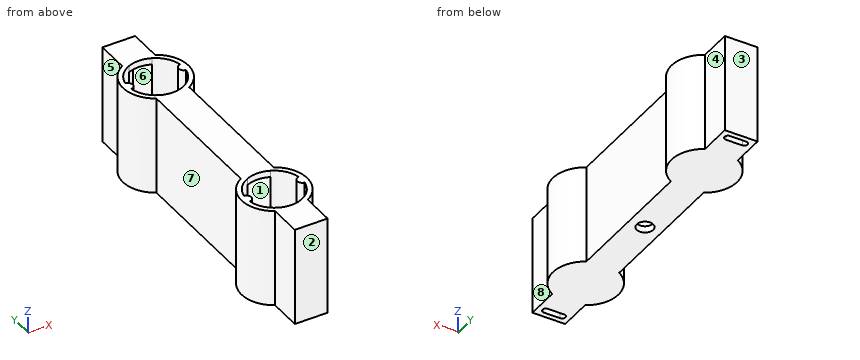
from build123d import *
from build123d.topology import SkipClean

# Parameters (mm, degrees)
BOSS_EXTRU_1_DEPTH      = 30
ENL_V_MAT_EXTRU_1_DEPTH = 28
BOSS_EXTRU_2_DEPTH      = 2
ESQUISSE5_R             = 2.5
ENL_V_MAT_EXTRU_2_DEPTH = 2
BOSS_EXTRU_3_DEPTH      = 29
ENL_V_MAT_EXTRU_4_DEPTH = 29
BOSS_EXTRU_4_DEPTH      = 28


with BuildPart() as part:
    # Esquisse1 → Boss.-Extru.1 (new body)
    with BuildSketch(Plane.XY):
        with BuildLine():
            Line((-5, -21.339745962), (-5, 21.339745962))
            ThreePointArc((-5, 21.339745962), (-10, 30), (-5, 38.660254038))
            Line((-5, 38.660254038), (-5, 48.660254038))
            Line((-5, 48.660254038), (5, 48.660254038))
            Line((5, 48.660254038), (5, 38.660254038))
            ThreePointArc((5, 38.660254038), (10, 30), (5, 21.339745962))
            Line((5, 21.339745962), (5, -21.339745962))
            ThreePointArc((5, -21.339745962), (10, -30), (5, -38.660254038))
            Line((5, -38.660254038), (5, -48.660254038))
            Line((5, -48.660254038), (-5, -48.660254038))
            Line((-5, -48.660254038), (-5, -38.660254038))
            ThreePointArc((-5, -38.660254038), (-10, -30), (-5, -21.339745962))
        make_face()
    extrude(amount=BOSS_EXTRU_1_DEPTH)

    # Esquisse2 → Enl_v. mat.-Extru.1 (cut)
    with BuildSketch(Plane.XY.offset(30)):
        with BuildLine():
            Line((-3.5, 22.254033308), (-3.5, -22.254033308))
            ThreePointArc((-3.5, -22.254033308), (-8.5, -30), (-3.5, -37.745966692))
            Line((-3.5, -37.745966692), (-3.5, -47.160254038))
            Line((-3.5, -47.160254038), (3.5, -47.160254038))
            Line((3.5, -47.160254038), (3.5, -37.745966692))
            ThreePointArc((3.5, -37.745966692), (8.5, -30), (3.5, -22.254033308))
            Line((3.5, -22.254033308), (3.5, 22.254033308))
            ThreePointArc((3.5, 22.254033308), (8.5, 30), (3.5, 37.745966692))
            Line((3.5, 37.745966692), (3.5, 47.160254038))
            Line((3.5, 47.160254038), (-3.5, 47.160254038))
            Line((-3.5, 47.160254038), (-3.5, 37.745966692))
            ThreePointArc((-3.5, 37.745966692), (-8.5, 30), (-3.5, 22.254033308))
        make_face()
    extrude(amount=-ENL_V_MAT_EXTRU_1_DEPTH, mode=Mode.SUBTRACT)

    # Esquisse3 → Boss.-Extru.2 (add)
    with SkipClean():  # keep this step's faces unmerged: merging them makes the solid invalid here
        with BuildSketch(Plane.XY.offset(30)):
            with BuildLine():
                Line((-3.5, 37.745966692), (-3.5, 47.160254038))
                Line((-3.5, 47.160254038), (3.5, 47.160254038))
                Line((3.5, 47.160254038), (3.5, 37.745966692))
                ThreePointArc((3.5, 37.745966692), (0, 38.5), (-3.5, 37.745966692))
            make_face()
            with BuildLine():
                Line((-3.5, -37.745966692), (-3.5, -47.160254038))
                Line((-3.5, -47.160254038), (3.5, -47.160254038))
                Line((3.5, -47.160254038), (3.5, -37.745966692))
                ThreePointArc((3.5, -37.745966692), (0, -38.5), (-3.5, -37.745966692))
            make_face()
            with BuildLine():
                Line((3.5, -22.254033308), (3.5, 22.254033308))
                ThreePointArc((3.5, 22.254033308), (0, 21.5), (-3.5, 22.254033308))
                Line((-3.5, 22.254033308), (-3.5, -22.254033308))
                ThreePointArc((-3.5, -22.254033308), (0, -21.5), (3.5, -22.254033308))
            make_face()
        extrude(amount=-BOSS_EXTRU_2_DEPTH)

    # Esquisse5 → Enl_v. mat.-Extru.2 (cut)
    with SkipClean():  # keep this step's faces unmerged: merging them makes the solid invalid here
        with BuildSketch(Plane(origin=(0, 0, 0), x_dir=(-1, 0, 0), z_dir=(0, 0, -1))):
            Circle(ESQUISSE5_R)
            with BuildLine():
                Line((2.5, 45.074057395), (-2.5, 45.074057395))
                ThreePointArc((-2.5, 45.074057395), (-3.5, 46.074057395), (-2.5, 47.074057395))
                Line((-2.5, 47.074057395), (2.5, 47.074057395))
                ThreePointArc((2.5, 47.074057395), (3.5, 46.074057395), (2.5, 45.074057395))
            make_face()
            with BuildLine():
                Line((2.5, -45.074057395), (-2.5, -45.074057395))
                ThreePointArc((-2.5, -45.074057395), (-3.5, -46.074057395), (-2.5, -47.074057395))
                Line((-2.5, -47.074057395), (2.5, -47.074057395))
                ThreePointArc((2.5, -47.074057395), (3.5, -46.074057395), (2.5, -45.074057395))
            make_face()
        extrude(amount=-ENL_V_MAT_EXTRU_2_DEPTH, mode=Mode.SUBTRACT)

    # Esquisse8 → Boss.-Extru.3 (add)
    with SkipClean():  # keep this step's faces unmerged: merging them makes the solid invalid here
        with BuildSketch(Plane.XY.offset(30)):
            with BuildLine():
                ThreePointArc((8.367647059, -28.50585051), (7, -30), (8.367647059, -31.49414949))
                ThreePointArc((8.367647059, -31.49414949), (0, -38.5), (-8.367647059, -31.49414949))
                ThreePointArc((-8.367647059, -31.49414949), (-7, -30), (-8.367647059, -28.50585051))
                ThreePointArc((-8.367647059, -28.50585051), (0, -21.5), (8.367647059, -28.50585051))
            make_face()
        extrude(amount=-BOSS_EXTRU_3_DEPTH)

    # Esquisse8_15 → Enl_v. mat.-Extru.4 (cut)
    with SkipClean():  # keep this step's faces unmerged: merging them makes the solid invalid here
        with BuildSketch(Plane.XY.offset(30)):
            with BuildLine():
                ThreePointArc((-3.5, -37.745966692), (0, -38.5), (3.5, -37.745966692))
                ThreePointArc((3.5, -37.745966692), (6.706829822, -35.221918588), (8.367647059, -31.49414949))
                ThreePointArc((8.367647059, -31.49414949), (7, -30), (8.367647059, -28.50585051))
                ThreePointArc((8.367647059, -28.50585051), (6.706829822, -24.778081412), (3.5, -22.254033308))
                ThreePointArc((3.5, -22.254033308), (0, -21.5), (-3.5, -22.254033308))
                ThreePointArc((-3.5, -22.254033308), (-6.706829822, -24.778081412), (-8.367647059, -28.50585051))
                ThreePointArc((-8.367647059, -28.50585051), (-7, -30), (-8.367647059, -31.49414949))
                ThreePointArc((-8.367647059, -31.49414949), (-6.706829822, -35.221918588), (-3.5, -37.745966692))
            make_face()
        extrude(amount=-ENL_V_MAT_EXTRU_4_DEPTH, mode=Mode.SUBTRACT)

    # Esquisse12 → Boss.-Extru.4 (add)
    with SkipClean():  # keep this step's faces unmerged: merging them makes the solid invalid here
        with BuildSketch(Plane.XY.offset(2)):
            with BuildLine():
                ThreePointArc((8.367647059, -31.49414949), (8.5, -30), (8.367647059, -28.50585051))
                ThreePointArc((8.367647059, -28.50585051), (7, -30), (8.367647059, -31.49414949))
            make_face()
            with BuildLine():
                ThreePointArc((-8.367647059, -31.49414949), (-7, -30), (-8.367647059, -28.50585051))
                ThreePointArc((-8.367647059, -28.50585051), (-8.5, -30), (-8.367647059, -31.49414949))
            make_face()
        boss_extru_4 = extrude(amount=BOSS_EXTRU_4_DEPTH)

    # Sym_trie1: Boss.-Extru.4 across plane
    with SkipClean():  # keep this step's faces unmerged: merging them makes the solid invalid here
        add(boss_extru_4.mirror(Plane.ZX))


solid = part.part
Source: CAD feature listing. Evaluate the final solid. Frame: model axes, mm. Face numbers are marked on the shaded views. A direction names the side the tool comes from. Round coordinates to 2 decimals unless told otherwise and drop trailing zeros. Loops run counter-clockwise (first coordinate to the right, second up) from the corner with the lowest first, then second, coordinate; pieces in that order, holes last. Notation, with made-up numbers: (-8.5, 67) - (17.5, 67) arc R17 cw to (17.5, 83) - close; hole circle Ø4 at (35, -2). An arc over 180 degrees is marked (long way). Write item = value, one per line. Start each with the question number.
Item 1: First-contact query: pin 1 Ø11 at (y, z) = (46, 17) entering from -X; pin 2 Ø10.5 at (y, z) = (-42, 13) entering from +X; pin 3 Ø9 at (y, z) = (-1.5, 22.5) entering from +X. Flat tips, straight axial feed; report the tip coordinate or a pass-through.
Item 2: Material intervals for line 1 (Y direction, x = 0, z = 0.95); line 2 (Y direction, x = 0, z = 1.5); line 3 (X direction, y = 20, z = 9), sorted ascending.
Item 3: Reachability of the marked faces 5, 6, 7 and 8 from +Z, -Z, +X, -X, +Y, -Y: full face, straight path, thin tool, end or side. Return the list, or none.
Item 4: Mould query, pull axis Y, two halves, no side actions, for the marked faces 1, 2, 3 and 4. Classes: released by +Y, released by -Y, zero draft, split by the parting line, or undercut.
Item 5: Section query D-D on y = -30.5. Output: boundary loops of the cut face in (x, z), plus the area to 3 significant figures.
Item 6: Section query B-B on y = 18.5. Output: boundary loops of the cut face in (x, z).
Item 7: Section query A-A on x = 0. Count the separate pieces of the cut face and the enclosed holes in it, plus the area to 3 significant figures.
Results list:
q1.pin_1 = -5
q1.pin_2 = 7.38
q1.pin_3 = 5
q2.line_1 = -48.66 to -47.07, -45.07 to -2.5, 2.5 to 45.07, 47.07 to 48.66
q2.line_2 = -48.66 to -47.07, -45.07 to -38.5, -21.5 to -2.5, 2.5 to 45.07, 47.07 to 48.66
q2.line_3 = -5 to -3.5, 3.5 to 5
q3.face_5 = +Z, -Z, -X, +Y
q3.face_6 = none
q3.face_7 = +Z, -Z, -X
q3.face_8 = +Z, -Z, +X, -Y
q4.face_1 = undercut
q4.face_2 = released by -Y
q4.face_3 = released by +Y
q4.face_4 = zero draft
q5.outline = (-9.99, 0) - (9.99, 0) - (9.99, 30) - (7.09, 30) - (7.09, 1) - (-7.09, 1) - (-7.09, 30) - (-9.99, 30) - close
q5.area = 188 mm²
q6.outline = (-5, 0) - (5, 0) - (5, 30) - (-5, 30) - close; hole (-3.5, 2) - (3.5, 2) - (3.5, 28) - (-3.5, 28) - close
q7.separate_pieces = 5
q7.enclosed_holes = 0
q7.area = 364 mm²
